The listing builds one solid part. Answer for the finished solid, in the listing's coordinates (mm). A direction names the side the tool comes from. Coordinates: 2 decimals unless noted, no trailing zeros. Order: outer loops, then holes, each group sorted by start corner. A loop starts at its lowest first (then second) coordinate and runs counter-clockwise, first axis right, second up. Notation, with made-up numbers: (-32, 35) -> (4, 35) arc R13 ccw to (4, 47) -> close; hole circle Ø10 at (-4.5, -2). An arc over 180 degrees is marked (long way). Write each question's results on one line, items separated by ' | '. Start each with the question number.
(1) The part is cut by section C-C, the plane z = -29. Give the vertices of the cut face in (x, y).
(2) The part is cut by section B-B, the plane x = 0. Give the vertices of the cut face in (y, z), then the cut area to 3 significant figures.
(3) Given pin 1 (6 mm diameter, centred on x = -32, y = 7.5, fed in from +Z); pin 2 (7.5 mm diameter, centred on y = 0, z = 0, fed in from -X); pin 3 (4 mm diameter, centred on y = 3.5, z = -48.5, fed in from +X); pin 4 (10 mm diameter, centred on x = -14, y = -8.5, fed in from -Z), each flat-ended and moving along its own axis, determine where each tip first touches the part or whether it passes through.
(4) Determine the mould class of faces 5 (the face through (-9, 4.4, 0.1)), 6 (the face through (0, -1, 24)), 7 (the face through (21, -1, -29)) for opening direction X: +X half, -X half, draft (parallel to the pull), parting line (faces both ways), or undercut.
(5) Straight lines are drawn through the part: L1, parallel to Z at x = 30, y = 0 (3 decimals); L2, parallel to Z at x = 0.5, y = 2.25; L3, parallel to Y at x = 27, z = 0 (3 decimals). For each, find the intervals that lie inside material, in ascending order.
(6) A tool of negligible diameter and unlimited length cuts with its end or side. For faces 1 (the face through (-25.56, -0.49, 18.38)), 2 (the face through (25.437, -0.875, -18.364)), 3 (the face through (-25.563, -0.875, -18.364)), 4 (the face through (0, -8, 0)), from which of +Z, -Z, +X, -X, +Y, -Y can it reach the whole face along a straight path? Write none if from no direction.
(7) The part is cut by section D-D, the plane z = -44. Give the vertices of the cut face in (x, y).
(8) The part is cut by section A-A, the plane y = 0. Give the vertices of the cut face in (x, z) (3 decimals), then the cut area to 3 significant figures.
```python
from build123d import *

# Parameters (mm, degrees)
BOSS_EXTRUDE1_DEPTH      = 12
BOSS_EXTRUDE1_DEPTH_BACK = 13
BOSS_EXTRUDE2_START      = -40
BOSS_EXTRUDE2_DEPTH      = 80
SKETCH2_W                = 18
SKETCH2_H                = 18
CUT_EXTRUDE1_DEPTH       = 20
CUT_EXTRUDE2_DEPTH       = 74.273460407
CUT_EXTRUDE2_DEPTH_BACK  = 74.273460407
SKETCH5_R                = 4.125
CHAMFER1_SIZE            = 10


# Read off the part's stored shape, not the designer's step: Boss-Extrude2
with BuildPart() as part:
    # Sketch1 → Boss-Extrude1 (new, two sides: drawn at the far end of the back side and taken through both)
    with BuildSketch(Plane(origin=(0, 0, 0), x_dir=(1, 0, 0), z_dir=(0, 1, 0)).offset(-BOSS_EXTRUDE1_DEPTH_BACK)):
        with BuildLine():
            Line((-21, -24), (21, -24))
            Line((21, -24), (21, 39))
            ThreePointArc((21, 39), (0, 60), (-21, 39))
            Line((-21, 39), (-21, -24))
        make_face()
    extrude(amount=BOSS_EXTRUDE1_DEPTH + BOSS_EXTRUDE1_DEPTH_BACK)

    # Boss-Extrude2 outline → Boss-Extrude2 (add)
    with BuildSketch(Plane(origin=(0, 0, 0), x_dir=(0, 0, -1), z_dir=(1, 0, 0)).offset(BOSS_EXTRUDE2_START)):
        with BuildLine():
            Line((-13, -13), (13, -13))
            ThreePointArc((13, -13), (18.372112666, -0.682258161), (13.928388277, 12))
            Line((13.928388277, 12), (-13.928388277, 12))
            ThreePointArc((-13.928388277, 12), (-18.372112666, -0.682258161), (-13, -13))
        make_face()
    extrude(amount=BOSS_EXTRUDE2_DEPTH)

    # Sketch2 → Cut-Extrude1 (cut)
    with BuildSketch(Plane(origin=(0, 12, 0), x_dir=(1, 0, 0), z_dir=(0, 1, 0))):
        Rectangle(SKETCH2_W, SKETCH2_H)
    extrude(amount=-CUT_EXTRUDE1_DEPTH, mode=Mode.SUBTRACT)

    # Sketch5 → Cut-Extrude2 (cut, two sides: drawn at the far end of the back side and taken through both)
    with BuildSketch(Plane(origin=(0, 0, 0), x_dir=(0, 0, -1), z_dir=(1, 0, 0)).offset(-CUT_EXTRUDE2_DEPTH_BACK)):
        Circle(SKETCH5_R)
    extrude(amount=CUT_EXTRUDE2_DEPTH + CUT_EXTRUDE2_DEPTH_BACK, mode=Mode.SUBTRACT)

    # Chamfer1
    # the kernel refuses this chamfer: 10 mm, written as the material it takes off along each edge
    with BuildSketch(Plane(origin=(40, 0, -1e-09), x_dir=(0, -0.8173943471187031, 0.5760785374394618), z_dir=(0, 0.5760785374394618, 0.8173943471187031))) as chamfer1_piece_1:
        Polygon((18.38477631 - CHAMFER1_SIZE, 0), (18.38477631, -CHAMFER1_SIZE), (18.38477631, 0), align=None)
    revolve(axis=Axis((40, 0, -1e-09), (1, 0, 0)), revolution_arc=246.096931862, mode=Mode.SUBTRACT)
    with BuildSketch(Plane(origin=(40, 0, 1e-09), x_dir=(0, 0.8578700425310862, -0.5138667046304052), z_dir=(0, -0.5138667046304052, -0.8578700425310862))) as chamfer1_piece_2:
        Polygon((18.38477631, -CHAMFER1_SIZE), (18.38477631 - CHAMFER1_SIZE, 0), (18.38477631, 0), align=None)
    revolve(axis=Axis((40, 0, 1e-09), (1, 0, 0)), revolution_arc=246.096931862, mode=Mode.SUBTRACT)
    with BuildSketch(Plane(origin=(-40, 0, 1e-09), x_dir=(0, 0.8578700425310862, -0.5138667046304052), z_dir=(0, -0.5138667046304052, -0.8578700425310862))) as chamfer1_piece_3:
        Polygon((18.38477631, CHAMFER1_SIZE), (18.38477631 - CHAMFER1_SIZE, 0), (18.38477631, 0), align=None)
    revolve(axis=Axis((-40, 0, 1e-09), (1, 0, 0)), revolution_arc=246.096931862, mode=Mode.SUBTRACT)
    with BuildSketch(Plane(origin=(-40, 0, -1e-09), x_dir=(0, -0.8173943471187031, 0.5760785374394618), z_dir=(0, 0.5760785374394618, 0.8173943471187031))) as chamfer1_piece_4:
        Polygon((18.38477631 - CHAMFER1_SIZE, 0), (18.38477631, CHAMFER1_SIZE), (18.38477631, 0), align=None)
    revolve(axis=Axis((-40, 0, -1e-09), (1, 0, 0)), revolution_arc=246.096931862, mode=Mode.SUBTRACT)


solid = part.part
```
Established:
1) outline: (-21, -13) -> (21, -13) -> (21, 12) -> (-21, 12) -> close
2) outline: (-13, -60) -> (12, -60) -> (12, -9) -> (-8, -9) -> (-8, 9) -> (12, 9) -> (12, 24) -> (-13, 24) -> close | area: 1,740 mm^2
3) pin 1: stops at z = 17.62 | pin 2: passes through | pin 3: stops at x = 19.62 | pin 4: stops at z = -57.97
4) face 5: undercut | face 6: draft | face 7: +X half
5) L1: z = -18.385 to -4.125, 4.125 to 18.385 | L2: z = -59.99 to -9, 9 to 24 | L3: y = -13 to -4.125, 4.125 to 12
6) face 1: +Z, -X | face 2: -Z, +X | face 3: -Z, -X | face 4: +Y
7) outline: (-20.4, -13) -> (20.4, -13) -> (20.4, 12) -> (-20.4, 12) -> close
8) outline: (-40, -8.385) -> (-30, -18.385) -> (-21, -18.385) -> (-21, -39) arc R21 ccw to (21, -39) -> (21, -18.385) -> (30, -18.385) -> (40, -8.385) -> (40, -4.125) -> (9, -4.125) -> (9, -9) -> (-9, -9) -> (-9, -4.125) -> (-40, -4.125) -> close; (-40, 4.125) -> (-9, 4.125) -> (-9, 9) -> (9, 9) -> (9, 4.125) -> (40, 4.125) -> (40, 8.385) -> (30, 18.385) -> (21, 18.385) -> (21, 24) -> (-21, 24) -> (-21, 18.385) -> (-30, 18.385) -> (-40, 8.385) -> close | area: 3,700 mm^2
